Verification items for the finished model (mm, model axes). Coordinates: 2 decimals unless noted, no trailing zeros. Order: outer loops, then holes, each group sorted by start corner. A loop starts at its lowest first (then second) coordinate and runs counter-clockwise, first axis right, second up. Notation, with made-up numbers: (49, 72) -> (63, 72) arc R14 cw to (63, 86) -> close; hole circle Ø11 at (5, 34.5). An arc over 180 degrees is marked (long way). Answer as CSV lines item,"result".
```python
from build123d import *

# Parameters (mm, degrees)
CYLINDER001_R     = 30
CYLINDER001_DEPTH = 75
CYLINDER_R        = 35
CYLINDER_DEPTH    = 75
FILLET_R          = 1.5


with BuildPart() as cylinder001:
    # Cylinder001 → Cylinder001 (new body)
    with BuildSketch(Plane.XY.offset(37)):
        Circle(CYLINDER001_R)
    extrude(amount=CYLINDER001_DEPTH)


with BuildPart() as fusion:
    # Sphere → Sphere (revolve)
    with BuildSketch(Plane(origin=(0, 0, 37), x_dir=(1, 0, 0), z_dir=(0, -1, 0))):
        with BuildLine():
            ThreePointArc((0, -30), (30, 0), (0, 30))
            Line((0, 30), (0, -30))
        make_face()
    revolve(axis=Axis((0, 0, 37), (0, 0, 1)))

    # Fusion: union Cylinder001
    add(cylinder001.part)


with BuildPart() as fillet_body:
    # Cylinder → Cylinder (new body)
    with BuildSketch(Plane.XY):
        Circle(CYLINDER_R)
    extrude(amount=CYLINDER_DEPTH)

    # Cut: cut Fusion
    add(fusion.part, mode=Mode.SUBTRACT)

    # Fillet
    fillet_edges = [fillet_body.edges().sort_by_distance(p)[0] for p in [
        (-35, 0, 0),
        (-35, 0, 75),
        (-30, 0, 75),
    ]]
    fillet(fillet_edges, radius=FILLET_R)


solid = fillet_body.part
```
Item 1: Section check C-C, the plane z = 51. Record the boundary of the cut face in (x, y), plus the area to 3 significant figures.
Answer list:
outline,"circle Ø70 at (0, 0); hole circle Ø60 at (0, 0)"
area,"1,020 mm2"
Item 2: Thickness scan on line 1 (Y direction, x = 0, z = 55.5); line 2 (Y direction, x = -8.5, z = 62); line 3 (X direction, y = -21.5, z = 53.5). Record the ranges inside material, lowest first.
Answer list:
line 1,"-35 to -30, 30 to 35"
line 2,"-33.95 to -28.77, 28.77 to 33.95"
line 3,"-27.62 to -20.92, 20.92 to 27.62"
Item 3: Depth check by flat-ended pin: pin 1 Ø10 at (x, z) = (27, 64) entering from -Y; pin 2 Ø1 at (x, z) = (-12.5, 12.5) entering from +Y; pin 3 Ø4 at (y, z) = (10.5, 8.5) entering from -X; pin 4 Ø12 at (y, z) = (4.5, 16.5) entering from -X. Enter the tip coordinate at first touch or a pass-through.
Answer list:
pin 1,"y = -27.22"
pin 2,"y = 32.88"
pin 3,"x = -33.95"
pin 4,"x = -35"
Item 4: Section check D-D, the plane z = 35.5. Record the boundary of the cut face in (x, y), plus the area to 3 significant figures.
Answer list:
outline,"circle Ø70 at (0, 0); hole circle Ø59.92 at (0, 0)"
area,"1,030 mm2"
Item 5: Section check A-A, the plane x = 0. Record the boundary of the cut face in (y, z).
Answer list:
outline,"(-35, 1.5) arc R1.5 ccw to (-33.5, 0) -> (33.5, 0) arc R1.5 ccw to (35, 1.5) -> (35, 73.5) arc R1.5 ccw to (33.5, 75) -> (31.5, 75) arc R1.5 ccw to (30, 73.5) -> (30, 37) arc R30 cw to (-30, 37) -> (-30, 73.5) arc R1.5 ccw to (-31.5, 75) -> (-33.5, 75) arc R1.5 ccw to (-35, 73.5) -> close"
Item 6: Release check for a two-part mould opening along X. For faces 1 (the cylindrical face through (-29.97, 1.32, 54.99)), 2 (the flat face through (0, 0, 0)), 3 (the cylindrical face through (-28, -21, 37)) record: +X half, -X half, draft (parallel to the pull), parting line (faces both ways), or undercut.
Answer list:
face 1,"undercut"
face 2,"draft"
face 3,"parting line"
